Verification items for the finished model (mm, model axes). A direction names the side the tool comes from. Round coordinates to 2 decimals unless told otherwise and drop trailing zeros. Write each loop counter-clockwise with the first axis right and the second up, starting at its lowest first coordinate (ties: lowest second). Pieces come first, ordered by that corner, then holes. Notation, with made-up numbers: (9.25, 56) - (34.25, 56) arc R16 cw to (34.25, 65) - close; hole circle Ø5 at (22, -30). An arc over 180 degrees is marked (long way). Write each question's results on one line, items separated by ' | '.
```python
from build123d import *

# Parameters (mm, degrees)
SKETCH_1_W      = 7
SKETCH_1_H      = 7
EXTRUDE_1_DEPTH = 7.1
SKETCH_2_W      = 3.9
SKETCH_2_H      = 3.9
EXTRUDE_2_DEPTH = 2.8
SKETCH_3_R      = 0.5
EXTRUDE_3_DEPTH = 3.6
SKETCH_4_W      = 3
SKETCH_4_H      = 2
EXTRUDE_4_DEPTH = 2.4


with BuildPart() as part:
    # 草图1 → 凸台-拉伸1 (new body)
    with BuildSketch(Plane(origin=(0, 0, 0), x_dir=(1, 0, 0), z_dir=(0, 1, 0))):
        with Locations((3.5, 3.5)):
            Rectangle(SKETCH_1_W, SKETCH_1_H)
    extrude(amount=EXTRUDE_1_DEPTH)

    # 草图2 → 凸台-拉伸2 (add)
    with BuildSketch(Plane(origin=(0, 7.1, 0), x_dir=(1, 0, 0), z_dir=(0, 1, 0))):
        with Locations((3.5, 3.5)):
            Rectangle(SKETCH_2_W, SKETCH_2_H)
    extrude(amount=EXTRUDE_2_DEPTH)

    # 草图3 → 凸台-拉伸3 (add)
    with BuildSketch(Plane.XZ):
        with Locations(Location((1.25, -1.5, 0), (0, 0, 270))):
            Circle(SKETCH_3_R)
        with Locations(Location((5.75, -1.5, 0), (0, 0, 270))):
            Circle(SKETCH_3_R)
        with Locations(Location((5.75, -5.5, 0), (0, 0, 270))):
            Circle(SKETCH_3_R)
        with Locations(Location((1.25, -5.5, 0), (0, 0, 270))):
            Circle(SKETCH_3_R)
    extrude(amount=EXTRUDE_3_DEPTH)

    # 草图4 → 凸台-拉伸4 (add)
    with BuildSketch(Plane(origin=(0, 9.9, 0), x_dir=(1, 0, 0), z_dir=(0, 1, 0))):
        with Locations((3.5, 3.5)):
            Rectangle(SKETCH_4_W, SKETCH_4_H)
    extrude(amount=EXTRUDE_4_DEPTH)


solid = part.part
```
(1) Section check D-D (y = 10.5). Record the cut outline in (x, z).
Answer:
outline: (2, -4.5) - (5, -4.5) - (5, -2.5) - (2, -2.5) - close
(2) Section check C-C (y = -2.25). Record the cut outline in (x, z), plus the area to 3 significant figures.
Answer:
outline: circle Ø1 at (1.25, -5.5); circle Ø1 at (1.25, -1.5); circle Ø1 at (5.75, -5.5); circle Ø1 at (5.75, -1.5) | area: 3.14 mm2
(3) Mould release check, pull along Z, two halves, no side actions. Record for faces 5 (the cylindrical face through (5.45, -1.77, -1.1)), 6 (the flat face through (3, 11, -2.5)), 7 (the flat face through (1.55, 8, -3)): released by +Z, released by -Z, zero draft, split by the parting line, or undercut.
Answer:
face 5: undercut | face 6: released by +Z | face 7: zero draft
(4) Go/stop test with flat-tipped pins: pin 1 Ø0.6 at (y, z) = (11, -3.5) entering from +X; pin 2 Ø1 at (y, z) = (8, -5.5) entering from +X; pin 3 Ø2 at (y, z) = (11.5, -3) entering from -X; pin 4 Ø3.5 at (x, z) = (4.5, -3) entering from -Y. Record where each tip stops, or that it passes through.
Answer:
pin 1: x = 5 | pin 2: x = 5.45 | pin 3: x = 2 | pin 4: y = -3.6
(5) Section check A-A (z = -4.75). Record the cut outline in (x, y), plus the area to 3 significant figures.
Answer:
outline: (0, 0) - (7, 0) - (7, 7.1) - (5.45, 7.1) - (5.45, 9.9) - (1.55, 9.9) - (1.55, 7.1) - (0, 7.1) - close | area: 60.6 mm2
(6) Thickness scan on L1, parallel to Y at x = 1.75, z = -2.75; L2, parallel to Y at x = 1, z = -4.5; L3, parallel to Z at x = 4, y = 9.25. Record the ranges inside material, lowest first.
Answer:
L1: 0 to 9.9 | L2: 0 to 7.1 | L3: -5.45 to -1.55
(7) Section check B-B (x = 5.75). Record the cut outline in (y, z), plus the area to 3 significant figures.
Answer:
outline: (-3.6, -6) - (0, -6) - (0, -7) - (7.1, -7) - (7.1, 0) - (0, 0) - (0, -1) - (-3.6, -1) - (-3.6, -2) - (0, -2) - (0, -5) - (-3.6, -5) - close | area: 56.9 mm2
(8) Set-up check for faces 1 (the flat face through (3, 8, -5.45)), 2 (the flat face through (3, 8, -1.55)), 3 (the flat face through (5.45, 8, -3)), 4 (the cylindrical face through (1.588, -1.775, -1.131)): record each of +Z, -Z, +X, -X, +Y, -Y from which the full face is reachable in a straight line by a thin tool's end or side.
Answer:
face 1: -Z, +X, -X, +Y | face 2: +Z, +X, -X, +Y | face 3: +Z, -Z, +X, +Y | face 4: -Y
